Could you check a few things on this drawing? It's one solid part, dimensions in mm from its lowest x, y, z. A direction names the side the tool comes from. Give positions to 0.01 mm unless a question says otherwise; leave off trailing zeros. Write each loop counter-clockwise with the first axis right and the second up, starting at its lowest first coordinate (ties: lowest second). Pieces come first, ordered by that corner, then holes. Notation, with made-up numbers: M 58.25,-6 L 106.25,-6 A10 ccw 106.25,13 Z; hole C -35.75,84 d3. An arc over 180 degrees is marked long. Answer as CSV lines item,"result". Start each with the question number.
Q1. Suppose I cut it at D-D (y = 10.5). Write out the boundary of the cut face in (x, z), then the cut area to 4 significant figures.
Q2. Thinking about a two-plate mould opening in Y: for the marked faces 3, 4 and 5, which applies, +Y half, -Y half, draft (parallel to the pull), parting line (faces both ways), or undercut?
Q3. Suppose I cut it at A-A (y = 16.4). Write out the boundary of the cut face in (x, z).
Q4. Suppose I cut it at B-B (x = 3). Write out the boundary of the cut face in (y, z).
Q5. For pin 1 (1 mm diameter, centred on x = 2, y = 5.5, fed in from +Z); pin 2 (5 mm diameter, centred on y = 9, z = 9.5, fed in from -X), each with a flat end and sliding along its axis, tell me the tip position at first contact or that it passes through.
Q6. Suppose I cut it at C-C (z = 18.25). Write out the boundary of the cut face in (x, y), then the cut area to 3 significant figures.
Q7. If I drill on line 1 along Y through (x, z) = (3, 5.5); line 2 along Z through (x, y) = (0.75, 10.5); line 3 along Y through (x, z) = (2.6, 6.25), over which ranges is the centre line in solid material (lowest first)?
Q8. On a 3-axis mill with a long thin cutter (end or side, diameter ignored), from which of +Z, -Z, +X, -X, +Y, -Y can I reach the whole of each face in a straight line? I mean the marked faces 1 and 2. Say none if no direction works.
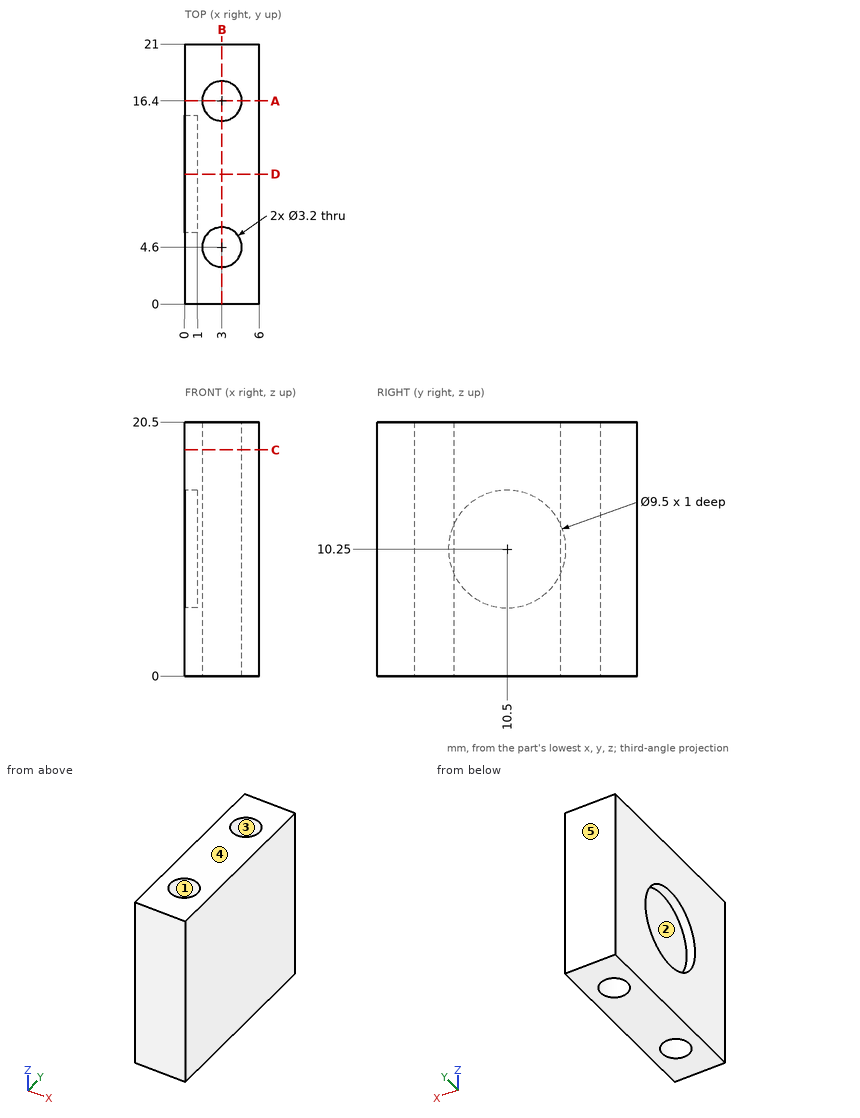
Resolved:
1,outline,"M 0,0 L 6,0 L 6,20.5 L 0,20.5 L 0,15 L 1,15 L 1,5.5 L 0,5.5 Z"
1,area,"113.5 mm^2"
2,face 3,"undercut"
2,face 4,"draft"
2,face 5,"+Y half"
3,outline,"M 0,0 L 1.4,0 L 1.4,20.5 L 0,20.5 Z; M 4.6,0 L 6,0 L 6,20.5 L 4.6,20.5 Z"
4,outline,"M 0,0 L 3,0 L 3,20.5 L 0,20.5 Z; M 6.2,0 L 14.8,0 L 14.8,20.5 L 6.2,20.5 Z; M 18,0 L 21,0 L 21,20.5 L 18,20.5 Z"
5,pin 1,"z = 20.5"
5,pin 2,"x = 1"
6,outline,"M 0,0 L 6,0 L 6,21 L 0,21 Z; hole C 3,4.6 d3.2; hole C 3,16.4 d3.2"
6,area,"110 mm^2"
7,line 1,"0 to 3, 6.2 to 14.8, 18 to 21"
7,line 2,"0 to 5.5, 15 to 20.5"
7,line 3,"0 to 3.05, 6.15 to 14.85, 17.95 to 21"
8,face 1,"+Z, -Z"
8,face 2,"-X"
